The drawing under review shows one solid part. Ordinate dimensions are in mm from its lowest x, y, z. Give positions to 0.01 mm unless a question says otherwise; leave off trailing zeros. Write each loop counter-clockwise with the first axis right and the second up, starting at its lowest first coordinate (ties: lowest second). Pieces come first, ordered by that corner, then holes.
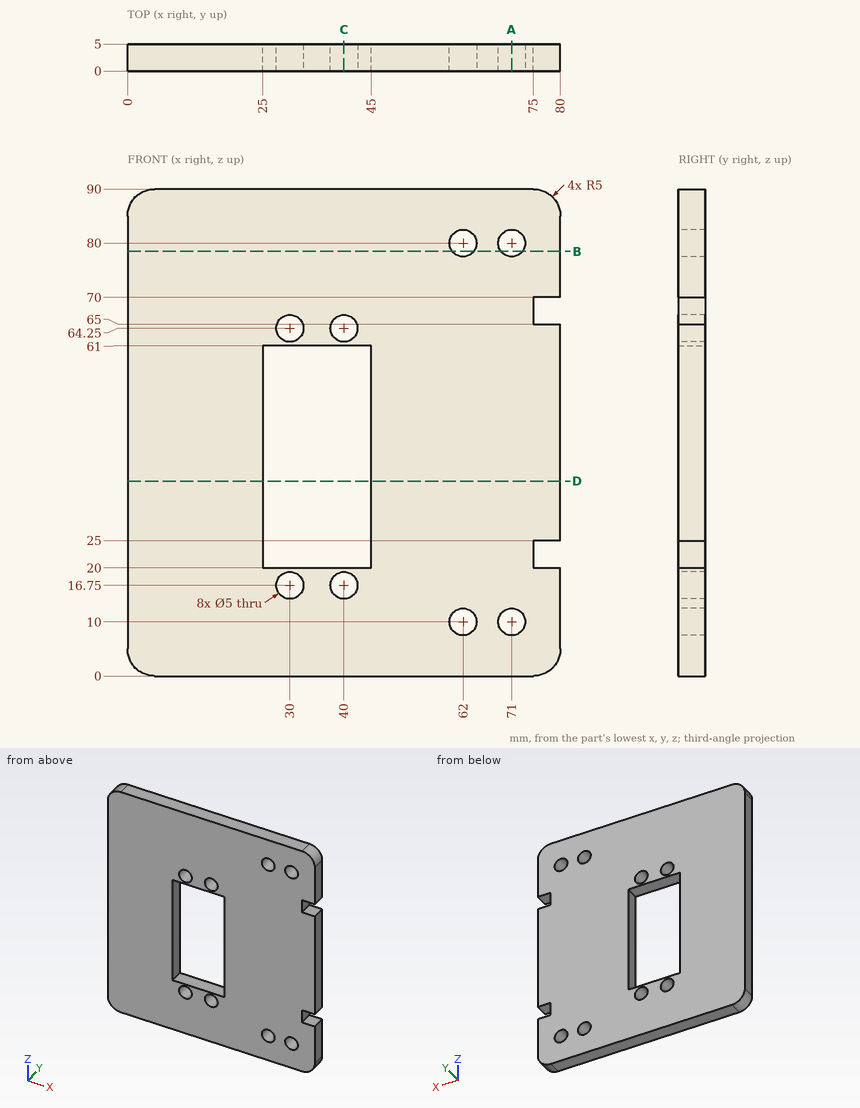
1) Consider section B-B, the plane z = 78.5. Give the boundary of the cut face in (x, y).
2) Consider section C-C, the plane x = 40. Give the boundary of the cut face in (y, z), then the cut area to 3 significant figures.
3) Consider section D-D, the plane z = 36. Give the boundary of the cut face in (x, y).
4) Consider section A-A, the plane x = 71. Give the boundary of the cut face in (y, z).
5) Insertion check: pin 1 (2.5 mm diameter, centred on x = 77, y = 2.5, fed in from +Z); pin 2 (2.5 mm diameter, centred on x = 78.5, y = 1.5, fed in from +Z); pin 3 (1.5 mm diameter, centred on y = 3.5, z = 66.5, fed in from +X). Each pin has a flat end and moves straight along its axis. Give the tip position at first contact, or say it passes through.
6) To check wall thickness, follow probe 1 along Z at (x, y) = (30, 3.45); probe 2 along Z at (x, y) = (62, 2.9); probe 3 along X at (y, z) = (3.45, 62.5). State the ranges of each line that lie inside material, in increasing order.
Answer block:
1. outline: (0, 0) - (60, 0) - (60, 5) - (0, 5) - close; (64, 0) - (69, 0) - (69, 5) - (64, 5) - close; (73, 0) - (80, 0) - (80, 5) - (73, 5) - close
2. outline: (0, 0) - (5, 0) - (5, 14.25) - (0, 14.25) - close; (0, 19.25) - (5, 19.25) - (5, 20) - (0, 20) - close; (0, 61) - (5, 61) - (5, 61.75) - (0, 61.75) - close; (0, 66.75) - (5, 66.75) - (5, 90) - (0, 90) - close
2. area: 195 mm2
3. outline: (0, 0) - (25, 0) - (25, 5) - (0, 5) - close; (45, 0) - (80, 0) - (80, 5) - (45, 5) - close
4. outline: (0, 0) - (5, 0) - (5, 7.5) - (0, 7.5) - close; (0, 12.5) - (5, 12.5) - (5, 77.5) - (0, 77.5) - close; (0, 82.5) - (5, 82.5) - (5, 90) - (0, 90) - close
5. pin 1: stops at z = 89.94
5. pin 2: stops at z = 89.47
5. pin 3: stops at x = 75
6. probe 1: z = 0 to 14.25, 19.25 to 20, 61 to 61.75, 66.75 to 90
6. probe 2: z = 0 to 7.5, 12.5 to 77.5, 82.5 to 90
6. probe 3: x = 0 to 28.21, 31.79 to 38.21, 41.79 to 80
